Could you check a few things on this drawing? It's one solid part, dimensions in mm from its lowest x, y, z. Give positions to 0.01 mm unless a question says otherwise; leave off trailing zeros. Order: outer loops, then holes, each group sorted by start corner. A loop starts at its lowest first (then second) coordinate and runs counter-clockwise, first axis right, second up. Notation, with made-up numbers: (79, -13.5) - (106, -13.5) arc R21 ccw to (106, 10.5) - close; hole circle Ø10 at (-22.75, 5.5). An arc over 180 degrees is marked (long way). Return JSON: item names as keys, results as strings.
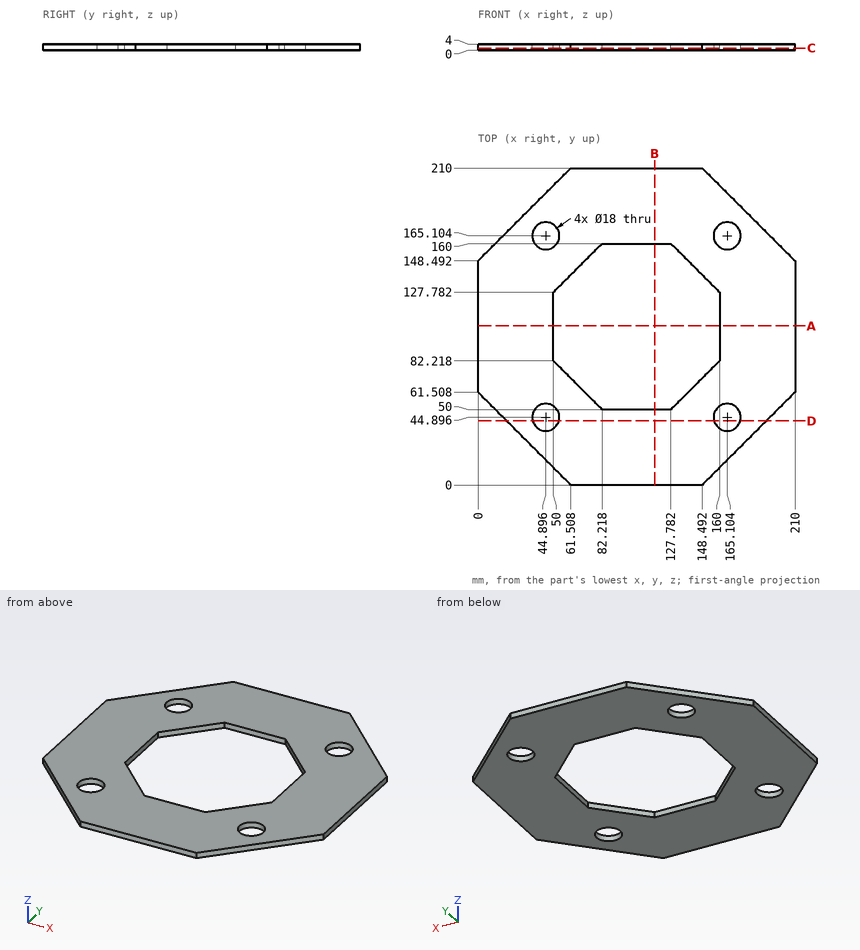
1. For pin 1 Ø16 at (x, y) = (44.9, 165.1) entering from +Z; pin 2 Ø1 at (x, z) = (32.5, 1.5) entering from +Y; pin 3 Ø1.5 at (y, z) = (60.5, 2.5) entering from -X, each with a flat end and sliding along its axis, tell me the tip position at first contact or that it passes through.
Checks:
{"pin 1": "through", "pin 2": "y = 181.49", "pin 3": "x = 0.26"}
2. If I drill on L1, parallel to Y at x = 127, z = 0.35; L2, parallel to X at y = 39, z = 1.4 (1 decimal), over which ranges is the centre line in solid material (lowest first)? Write a range as [from, to].
Checks:
{"L1": "[0, 50], [160, 210]", "L2": "[22.5, 38.1], [51.7, 158.3], [171.9, 187.5]"}
3. Suppose I cut it at D-D (y = 42.5). List the corners of the cut face in (x, z) for me.
Checks:
{"outline": "(19.01, 0) - (36.22, 0) - (36.22, 4) - (19.01, 4) - close; (53.57, 0) - (156.43, 0) - (156.43, 4) - (53.57, 4) - close; (173.78, 0) - (190.99, 0) - (190.99, 4) - (173.78, 4) - close"}
4. Suppose I cut it at C-C (z = 1.25). List the corners of the cut face in (x, y) for me, plus the area to 3 significant figures.
Checks:
{"outline": "(0, 61.51) - (61.51, 0) - (148.49, 0) - (210, 61.51) - (210, 148.49) - (148.49, 210) - (61.51, 210) - (0, 148.49) - close; hole circle Ø18 at (44.9, 44.9); hole circle Ø18 at (44.9, 165.1); hole (50, 82.22) - (82.22, 50) - (127.78, 50) - (160, 82.22) - (160, 127.78) - (127.78, 160) - (82.22, 160) - (50, 127.78) - close; hole circle Ø18 at (165.1, 44.9); hole circle Ø18 at (165.1, 165.1)", "area": "25,500 mm^2"}
5. Suppose I cut it at A-A (y = 105.5). List the corners of the cut face in (x, z) for me.
Checks:
{"outline": "(0, 0) - (50, 0) - (50, 4) - (0, 4) - close; (160, 0) - (210, 0) - (210, 4) - (160, 4) - close"}
